Could you check a few things on this model? Use its own coordinates, in mm. A direction names the side the tool comes from. Give positions to 0.01 mm unless a question says otherwise; leave off trailing zeros. Write each loop counter-clockwise with the first axis right and the second up, starting at its lowest first coordinate (ties: lowest second). Pieces come first, ordered by that corner, then holes. Notation, with made-up numbers: M 69.5,41.5 L 123.5,41.5 A21 cw 123.5,52.5 Z; hole C 13,39.25 d7. An arc over 180 degrees is marked long. Use one line per item in the form item = value.
from build123d import *

# Parameters (mm, degrees)
ESQUISSE1_R      = 20
EXTRUSION1_DEPTH = 44
ESQUISSE2_R      = 19
EXTRUSION2_DEPTH = 18.8
ESQUISSE3_W      = 38
ESQUISSE3_H      = 38
EXTRUSION3_DEPTH = 4.4
ESQUISSE4_R      = 1.25
EXTRUSION4_DEPTH = 73.909807296
ESQUISSE5_R      = 6
EXTRUSION5_DEPTH = 6.55
ESQUISSE6_R      = 3
EXTRUSION6_DEPTH = 15.45


with BuildPart() as part:
    # Esquisse1 → Extrusion1 (new body)
    with BuildSketch(Plane.XY):
        Circle(ESQUISSE1_R)
    extrude(amount=EXTRUSION1_DEPTH)

    # Esquisse2 → Extrusion2 (add)
    with BuildSketch(Plane.XY.offset(44)):
        Circle(ESQUISSE2_R)
    extrude(amount=EXTRUSION2_DEPTH)

    # Esquisse3 → Extrusion3 (add)
    with BuildSketch(Plane.XY.offset(62.8)):
        Rectangle(ESQUISSE3_W, ESQUISSE3_H)
    extrude(amount=EXTRUSION3_DEPTH)

    # Esquisse4 → Extrusion4 (cut, through all)
    with BuildSketch(Plane.XY.offset(67.2)):
        with Locations((-15.25, 15.25)):
            Circle(ESQUISSE4_R)
        with Locations((15.25, 15.25)):
            Circle(ESQUISSE4_R)
        with Locations((15.25, -15.25)):
            Circle(ESQUISSE4_R)
        with Locations((-15.25, -15.25)):
            Circle(ESQUISSE4_R)
    extrude(amount=-EXTRUSION4_DEPTH, mode=Mode.SUBTRACT)

    # Esquisse5 → Extrusion5 (add)
    with BuildSketch(Plane.XY.offset(67.2)):
        with Locations((0, -9)):
            Circle(ESQUISSE5_R)
    extrude(amount=EXTRUSION5_DEPTH)

    # Esquisse6 → Extrusion6 (add)
    with BuildSketch(Plane.XY.offset(73.75)):
        with Locations((0, -9)):
            Circle(ESQUISSE6_R)
    extrude(amount=EXTRUSION6_DEPTH)


solid = part.part
1) For pin 1 Ø1.5 at (x, y) = (8.5, 0.5) entering from +Z; pin 2 Ø3.5 at (x, z) = (4.5, 65) entering from -Y; pin 3 Ø1.3 at (x, z) = (-3.5, 65.5) entering from +Y, each with a flat end and sliding along its axis, tell me the tip position at first contact or that it passes through.
Checked values:
pin_1 = 67.2
pin_2 = -19
pin_3 = 19
2) If I drill on L1, parallel to Y at x = 15.25, z = 65.2; L2, parallel to Z at x = -18, y = 6.5; L3, parallel to Z at x = 0, y = 4, over which ranges is the centre line in solid material (lowest first)?
Checked values:
L1 = -19 to -16.5, -14 to 14, 16.5 to 19
L2 = 0 to 44, 62.8 to 67.2
L3 = 0 to 67.2
3) I want a section at D-D, the plane x = 12. Please give me the cut outline in (y, z).
Checked values:
outline = M -19,62.8 L -14.73,62.8 L -14.73,44 L -16,44 L -16,0 L 16,0 L 16,44 L 14.73,44 L 14.73,62.8 L 19,62.8 L 19,67.2 L -19,67.2 Z
4) I want a section at C-C, the plane y = 8. Please give me the cut outline in (x, z), plus the area to 3 significant figures.
Checked values:
outline = M -19,62.8 L -17.23,62.8 L -17.23,44 L -18.33,44 L -18.33,0 L 18.33,0 L 18.33,44 L 17.23,44 L 17.23,62.8 L 19,62.8 L 19,67.2 L -19,67.2 Z
area = 2,430 mm2
5) For faces 1 (the flat face through (-13.8, -15.1, 62.8)), 2 (the flat face through (1, -6, 73.75)), 3 (the flat face through (13.7, -15.1, 62.8)), 4 (the flat face through (0, 19, 65)), which set-ups out of +Z, -Z, +X, -X, +Y, -Y let a thin tool reach every point of the face, with its end or its side?
Checked values:
face_1 = -X, -Y
face_2 = +Z
face_3 = +X, -Y
face_4 = +Z, +X, -X, +Y
6) Thinking about a two-plate mould opening in Y: for faces 5 (the cylindrical face through (8.767, -16.856, 53.268)), 6 (the cylindrical face through (14.329, 16.095, 65.031)), 7 (the flat face through (-14, 14, 62.8)), 8 (the cylindrical face through (-15.41, -14.01, 65.03)), which applies, released by +Y, released by -Y, zero draft, split by the parting line, or undercut?
Checked values:
face_5 = split by the parting line
face_6 = undercut
face_7 = zero draft
face_8 = undercut
7) I want a section at A-A, the plane x = -15.25. Please give me the cut outline in (y, z), plus the area to 3 significant figures.
Checked values:
outline = M -19,62.8 L -16.5,62.8 L -16.5,67.2 L -19,67.2 Z; M -14,62.8 L -11.33,62.8 L -11.33,44 L -12.94,44 L -12.94,0 L 12.94,0 L 12.94,44 L 11.33,44 L 11.33,62.8 L 14,62.8 L 14,67.2 L -14,67.2 Z; M 16.5,62.8 L 19,62.8 L 19,67.2 L 16.5,67.2 Z
area = 1,710 mm2
